Part model, mm, in its own coordinate system. A direction names the side the tool comes from. Round coordinates to 2 decimals unless told otherwise and drop trailing zeros. Loops run counter-clockwise (first coordinate to the right, second up) from the corner with the lowest first, then second, coordinate; pieces in that order, holes last.
(1) Tool access for faces 4 (the face through (-216.727, 39.979, 2.88)), 5 (the face through (-131.09, 167.41, 2.96)): list every direction of +Z, -Z, +X, -X, +Y, -Y with a clear straight run to the whole face (end or side of a thin tool).
(2) Cut at C-C on x = -211.5. List the corners of the cut face in (y, z), then the cut area to 3 significant figures.
(3) Cut at A-A on x = -50.8. List the corners of the cut face in (y, z), then the cut area to 3 significant figures.
(4) Mould opens along Y. For faces 1 (the face through (3.66, -10.2, 2.88)), 2 (the face through (-153, 93, 5.842)), 3 (the face through (-109.6, 85.7, 3)) say: +Y half, -Y half, draft (parallel to the pull), parting line (faces both ways), or undercut.
(5) Cut at B-B on z = 3.65. List the corners of the cut face in (x, y) (1 decimal).
(6) Probe probe 1 along X at (y, z) = (20, 4.45); probe 2 along X at (y, z) = (-11, 3.2); probe 3 along X at (y, z) = (36.5, 2.95). List the from-to ranges inside material, lowest first.
(7) Flat gauge pins, fed straight in: pin 1 (1 mm diameter, centred on y = 116.5, z = 1, fed in from +X); pin 2 (23 mm diameter, centred on x = -130.99, y = 146.51, fed in from +Z); pin 3 (2 mm diameter, centred on y = 83, z = 5, fed in from +X); pin 4 (1.5 mm diameter, centred on x = -168, z = 3, fed in from -Y). Where does each tip first touch, or does it go through?
from build123d import *

# Parameters (mm, degrees)
SKETCH1_R           = 14.2875
BOSS_EXTRUDE1_DEPTH = 5.842
FILLET6_R           = 35.56
FILLET10_R          = 27.94
FILLET13_R          = 50.8


with BuildPart() as part:
    # Sketch1 → Boss-Extrude1 (new body)
    with BuildSketch(Plane(origin=(0, 0, 0), x_dir=(-1, 0, 0), z_dir=(0, 0, -1))):
        with BuildLine():
            Line((316.43857867, 42.94910124), (130.990896358, 174.671247093))
            Line((130.990896358, 174.671247093), (31.981087973, 112.057039535))
            Line((31.981087973, 112.057039535), (-15.378230565, 9.100654441))
            ThreePointArc((-15.378230565, 9.100654441), (-4.576133352, -23.72569398), (28.948253716, -15.337015504))
            Line((28.948253716, -15.337015504), (105.434059084, 104.999617888))
            Line((105.434059084, 104.999617888), (287.729052218, -1.503728312))
            ThreePointArc((287.729052218, -1.503728312), (323.338289689, 6.995643737), (316.43857867, 42.94910124))
        make_face()
        with Locations((301.089652101, 21.3647594)):
            Circle(SKETCH1_R, mode=Mode.SUBTRACT)
        with Locations((130.990896358, 146.510317071)):
            Circle(SKETCH1_R, mode=Mode.SUBTRACT)
        with Locations((50.8, 98.679)):
            Circle(SKETCH1_R, mode=Mode.SUBTRACT)
        with Locations((7.675076536, -1.503728312)):
            Circle(SKETCH1_R, mode=Mode.SUBTRACT)
    extrude(amount=-BOSS_EXTRUDE1_DEPTH)

    # Fillet6
    fillet6_edges = [part.edges().sort_by_distance(p)[0] for p in [
        (-130.990896358, 174.671247093, 2.921),
    ]]
    fillet(fillet6_edges, radius=FILLET6_R)

    # Fillet10
    fillet10_edges = [part.edges().sort_by_distance(p)[0] for p in [
        (-31.981087973, 112.057039535, 2.921),
    ]]
    fillet(fillet10_edges, radius=FILLET10_R)

    # Fillet13
    fillet13_edges = [part.edges().sort_by_distance(p)[0] for p in [
        (-105.434059084, 104.999617888, 2.921),
    ]]
    fillet(fillet13_edges, radius=FILLET13_R)


solid = part.part
Final values:
1. face 4: +Z, -Z, -Y
1. face 5: +Z, -Z, +Y
2. outline: (43.03, 0) - (117.49, 0) - (117.49, 5.84) - (43.03, 5.84) - close
2. area: 435 mm2
3. outline: (19.04, 0) - (84.39, 0) - (84.39, 5.84) - (19.04, 5.84) - close; (112.97, 0) - (123.96, 0) - (123.96, 5.84) - (112.97, 5.84) - close
3. area: 446 mm2
4. face 1: undercut
4. face 2: draft
4. face 3: -Y half
5. outline: (-316.4, 42.9) arc R26.5 ccw to (-287.7, -1.5) - (-147.7, 80.3) arc R50.8 cw to (-79.2, 63.7) - (-28.9, -15.3) arc R25.4 ccw to (15.4, 9.1) - (-28.5, 104.5) arc R27.9 ccw to (-39, 116.5) - (-110.8, 161.9) arc R35.6 ccw to (-150.4, 160.9) - close; hole circle Ø28.6 at (-301.1, 21.4); hole circle Ø28.6 at (-131, 146.5); hole circle Ø28.6 at (-50.8, 98.7); hole circle Ø28.6 at (-7.7, -1.5)
6. probe 1: x = -327.54 to -315.31, -286.87 to -250.92, -51.41 to 10.36
6. probe 2: x = -31.7 to -18.35, 3 to 15.86
6. probe 3: x = -322.82 to -222.68, -61.9 to 2.77
7. pin 1: stops at x = -38.24
7. pin 2: passes through
7. pin 3: stops at x = -18.16
7. pin 4: stops at y = 68.01
